from build123d import *

# Parameters (mm, degrees)
SKETCH_1_W               = 60
SKETCH_1_H               = 25
EXTRUDE_1_DEPTH          = 5
SKETCH_2_W               = 60
SKETCH_2_H               = 5
EXTRUDE_2_DEPTH          = 120
SKETCH_3_W               = 60
SKETCH_3_H               = 5
EXTRUDE_3_DEPTH          = 20
SKETCH_4_R               = 1.5
CUT_EXTRUDE_1_DEPTH      = 20
SKETCH_5_R               = 6.5
CUT_EXTRUDE_2_DEPTH      = 121
CUT_EXTRUDE_2_DEPTH_BACK = 6
SKETCH_6_R               = 3.5
CUT_EXTRUDE_3_DEPTH      = 121
CUT_EXTRUDE_3_DEPTH_BACK = 6


with BuildPart() as part:
    # 스케치1 → 보스-돌출1 (new body)
    with BuildSketch(Plane.XY):
        with Locations((30, 12.5)):
            Rectangle(SKETCH_1_W, SKETCH_1_H)
    extrude(amount=EXTRUDE_1_DEPTH)

    # 스케치2 → 보스-돌출2 (add)
    with BuildSketch(Plane(origin=(0, 0, 0), x_dir=(-1, 0, 0), z_dir=(0, 0, -1))):
        with Locations((-30, 2.5)):
            Rectangle(SKETCH_2_W, SKETCH_2_H)
    extrude(amount=EXTRUDE_2_DEPTH)

    # 스케치3 → 보스-돌출3 (add)
    with BuildSketch(Plane(origin=(0, 5, 0), x_dir=(1, 0, 0), z_dir=(0, 1, 0))):
        with Locations((30, 32.5)):
            Rectangle(SKETCH_3_W, SKETCH_3_H)
    extrude(amount=EXTRUDE_3_DEPTH)

    # 스케치4 → 컷-돌출1 (cut)
    with BuildSketch(Plane(origin=(0, 0, 0), x_dir=(-1, 0, 0), z_dir=(0, 0, -1))):
        with Locations((-57, 22)):
            Circle(SKETCH_4_R)
        with Locations((-57, 8)):
            Circle(SKETCH_4_R)
        with Locations((-3, 22)):
            Circle(SKETCH_4_R)
        with Locations((-3, 8)):
            Circle(SKETCH_4_R)
    extrude(amount=-CUT_EXTRUDE_1_DEPTH, mode=Mode.SUBTRACT)

    # 스케치5 → 컷-돌출2 (cut, two sides)
    with BuildSketch(Plane(origin=(0, 0, 0), x_dir=(-1, 0, 0), z_dir=(0, 0, -1))) as cut_extrude_2_sk:
        with Locations((-33.62939322, 15)):
            Circle(SKETCH_5_R)
        with Locations((-16.699372841, 15)):
            Circle(SKETCH_5_R)
    extrude(amount=CUT_EXTRUDE_2_DEPTH, mode=Mode.SUBTRACT)
    extrude(cut_extrude_2_sk.sketch, amount=-CUT_EXTRUDE_2_DEPTH_BACK, mode=Mode.SUBTRACT)

    # 스케치6 → 컷-돌출3 (cut, two sides)
    with BuildSketch(Plane(origin=(0, 0, 0), x_dir=(-1, 0, 0), z_dir=(0, 0, -1))) as cut_extrude_3_sk:
        with Locations((-47.855782548, 15)):
            Circle(SKETCH_6_R)
    extrude(amount=CUT_EXTRUDE_3_DEPTH, mode=Mode.SUBTRACT)
    extrude(cut_extrude_3_sk.sketch, amount=-CUT_EXTRUDE_3_DEPTH_BACK, mode=Mode.SUBTRACT)


solid = part.part
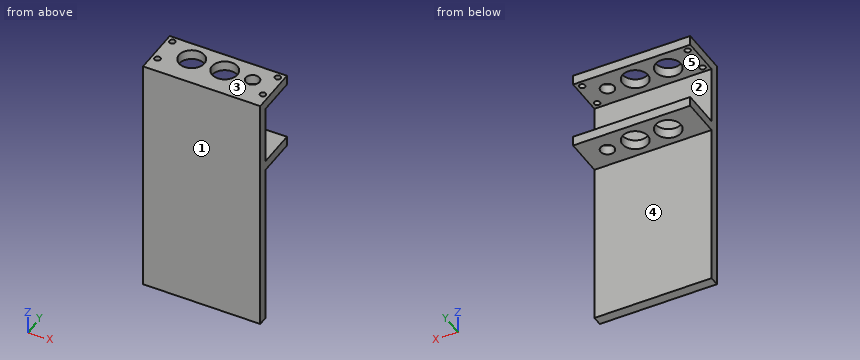
Work out the finished part from the listing and answer in its coordinate system (mm). Face numbers are marked on the shaded views. A direction names the side the tool comes from. Coordinates: 2 decimals unless noted, no trailing zeros. Order: outer loops, then holes, each group sorted by start corner. A loop starts at its lowest first (then second) coordinate and runs counter-clockwise, first axis right, second up. Notation, with made-up numbers: (5.5, 47.5) - (34.5, 47.5) arc R18 ccw to (34.5, 54.5) - close; hole circle Ø7 at (26, 19). An arc over 180 degrees is marked (long way). Put each result on its own line as item: value. Start each with the question number.
1) Find section D-D (z = -60). Give the vertices of the cut face in (x, y).
2) Find section C-C (x = 42). Give the vertices of the cut face in (y, z), plus the area to 3 significant figures.
3) Find section B-B (x = 3). Give the vertices of the cut face in (y, z).
4) For the marked faces 4 and 5, determine the directions among +Z, -Z, +X, -X, +Y, -Y from which every point of the face is accessible in a straight line to the end or side of a thin tool.
5) For a pull along Z with two mould halves and no side action, classify the marked faces 1, 2 and 3 as released by +Z, released by -Z, zero draft, split by the parting line, or undercut.
6) Find section A-A (y = 15). State how many separate pieces and enclosed holes the cut face has, plus the area to 3 significant figures.
7) Find the intervals of material crossed by line 1 (X direction, y = 15, z = -31.1); line 2 (Z direction, x = 22, y = 19.75); line 3 (Y direction, x = 3, z = 2.9), in increasing order. Write a range as from..to.
8) Flat-ended cylindrical pins translate along their axes: pin 1 (11.5 mm diameter, centred on x = 16.7, y = 15, fed in from +Z); pin 2 (3.5 mm diameter, centred on x = 3, y = 22, fed in from -Z); pin 3 (4 mm diameter, centred on x = 22, z = -17.5, fed in from +Y); pin 4 (6 mm diameter, centred on x = 30, y = 18.5, fed in from +Z). Find the tip coordinate at first contact, or state that the pin passes through.
Results list:
1. outline: (0, 0) - (60, 0) - (60, 5) - (0, 5) - close
2. outline: (0, -120) - (5, -120) - (5, -35) - (25, -35) - (25, -30) - (5, -30) - (5, 0) - (25, 0) - (25, 5) - (0, 5) - close
2. area: 825 mm^2
3. outline: (0, -120) - (5, -120) - (5, -35) - (25, -35) - (25, -30) - (5, -30) - (5, 0) - (6.5, 0) - (6.5, 5) - (0, 5) - close; (9.5, 0) - (20.5, 0) - (20.5, 5) - (9.5, 5) - close; (23.5, 0) - (25, 0) - (25, 5) - (23.5, 5) - close
4. face 4: -Z, +X, -X, +Y
4. face 5: +X, -X, +Y
5. face 1: zero draft
5. face 2: undercut
5. face 3: released by +Z
6. separate pieces: 8
6. enclosed holes: 0
6. area: 270 mm^2
7. line 1: x = 0..10.2, 23.2..27.13, 40.13..44.36, 51.36..60
7. line 2: z = -35..-30, 0..5
7. line 3: y = 0..6.5, 9.5..20.5, 23.5..25
8. pin 1: passes through
8. pin 2: stops at z = -35
8. pin 3: stops at y = 5
8. pin 4: stops at z = 5
